Part model, mm, in its own coordinate system. A direction names the side the tool comes from. Round coordinates to 2 decimals unless told otherwise and drop trailing zeros. Write each loop counter-clockwise with the first axis right and the second up, starting at its lowest first coordinate (ties: lowest second). Pieces come first, ordered by that corner, then holes.
```python
from build123d import *


with BuildPart() as f1:
    # F0 (on Front) → F1 (revolve)
    with BuildSketch(Plane.XZ):
        Polygon((24.926189, 75.470962), (0, 75.470962), (0, -75.470954), (40.648924, -75.470954), (40.648924, 43.620129), (33.977756, 47.164189), (39.69726, 57.930309), (24.926189, 65.777443), align=None)
    revolve(axis=Axis((0, 0, 4e-06), (0, 0, 1)))


solid = f1.part
```
Q1. Cut at C-C on z = -34.5. Write the cut outline in (x, y).
Values follow:
outline: circle Ø81.3 at (0, 0)
Q2. Mould opens along Z. For faces 4 (the conical face through (-7.44, -33.52, 47.84)), 5 (the flat face through (0, 0, 75.471)), 6 (the cylindrical face through (-8.812, -39.682, -15.092)) say: +Z half, -Z half, draft (parallel to the pull), parting line (faces both ways), or undercut.
Values follow:
face 4: undercut
face 5: +Z half
face 6: draft
Q3. Drop flat-ended pins along their axis: pin 1 (10 mm diameter, centred on x = -26, y = -25.5, fed in from +Z); pin 2 (1 mm diameter, centred on x = 27, z = -46.5, fed in from -Y); pin 3 (5 mm diameter, centred on x = -10.5, z = 55.5, fed in from +Y). Give the stop position or say it passes through.
Values follow:
pin 1: stops at z = 62.33
pin 2: stops at y = -30.82
pin 3: stops at y = 38.47
Q4. Cut at A-A on y = 0. Write the cut outline in (x, z), plus the area to 3 significant figures.
Values follow:
outline: (-40.65, -75.47) - (40.65, -75.47) - (40.65, 43.62) - (33.98, 47.16) - (39.7, 57.93) - (24.93, 65.78) - (24.93, 75.47) - (-24.93, 75.47) - (-24.93, 65.78) - (-39.7, 57.93) - (-33.98, 47.16) - (-40.65, 43.62) - close
area: 11,700 mm2
Q5. Which spindle directions (+Z, -Z, +X, -X, +Y, -Y) get a long thin tool onto all of the face, cutting with end or side? Do faces 1 (the cylindrical face through (23.025, -9.547, 70.692)), 2 (the flat face through (1, 1, -75.471)), 3 (the conical face through (-27.221, -20.872, 46.992)). Say none if no direction does.
Values follow:
face 1: +Z
face 2: -Z, +X, -X, +Y, -Y
face 3: none
Q6. Wall check: L1, parallel to Z at x = 24.5, y = -29; L2, parallel to Z at x = -26.5, y = -26.5; L3, parallel to Y at x = -31.5, z = 10.5. Give the ranges that are in metal, low to high.
Values follow:
L1: z = -75.47 to 45.05, 54.67 to 58.85
L2: z = -75.47 to 45.31, 53.75 to 59.11
L3: y = -25.69 to 25.69
